Check sheet for the modelled part. Datum: model origin and axes. Units: mm. A direction names the side the tool comes from. Give positions to 0.01 mm unless a question says otherwise; leave off trailing zeros. Write each loop counter-clockwise with the first axis right and the second up, starting at its lowest first coordinate (ties: lowest second). Pieces come first, ordered by that corner, then holes. Notation, with made-up numbers: (64.5, -0.75) - (118.5, -0.75) arc R27 cw to (118.5, 36.25) - close; hole circle Ø2 at (45.25, 27.25). An arc over 180 degrees is marked (long way). Return JSON: item names as keys, results as strings. Group by question number.
```python
from build123d import *

# Parameters (mm, degrees)
SKETCH_1_W           = 17
SKETCH_1_H           = 6
EXTRUDE_1_DEPTH      = 15
EXTRUDE_2_DEPTH      = 6
EXTRUDE_2_DEPTH_BACK = 6
FILLET_4_R           = 1
FILLET_5_R           = 1
FILLET_6_R           = 1


with BuildPart() as part:
    # Эскиз1 → Бобышка-Вытянуть1 (new body)
    with BuildSketch(Plane.XY):
        with BuildLine():
            Line((30, 0), (-30, 0))
            ThreePointArc((-30, 0), (0, -30), (30, 0))
        make_face()
        with Locations((0, -12.426630435)):
            Rectangle(SKETCH_1_W, SKETCH_1_H, mode=Mode.SUBTRACT)
    extrude(amount=EXTRUDE_1_DEPTH)

    # Эскиз6 → Бобышка-Вытянуть2 (add, two sides: drawn at the far end of the back side and taken through both)
    with BuildSketch(Plane(origin=(0, 0, 0), x_dir=(0, 0, -1), z_dir=(1, 0, 0)).offset(-EXTRUDE_2_DEPTH_BACK)):
        Polygon((-14.990436671, -0.00212283), (-14.990436671, 17.99787717), (10.009563329, 17.99787717), (10.009563329, 11.99787717), (-8.498173606, 11.99787717), (-8.498173606, -0.00212283), align=None)
    extrude(amount=EXTRUDE_2_DEPTH + EXTRUDE_2_DEPTH_BACK)

    # Скругление4
    fillet_4_edges = [part.edges().sort_by_distance(p)[0] for p in [
        (-6, 8.998938585, 14.990436671),
    ]]
    fillet(fillet_4_edges, radius=FILLET_4_R)

    # Скругление5
    fillet_5_edges = [part.edges().sort_by_distance(p)[0] for p in [
        (6, 8.998938585, 14.990436671),
        (6, 17.99787717, 2.490436671),
        (-6, 17.99787717, 1.990436671),
        (0.5, 17.99787717, 14.990436671),
        (-5.707106781, 17.99787717, 14.697543453),
    ]]
    fillet(fillet_5_edges, radius=FILLET_5_R)

    # Скругление6
    fillet_6_edges = [part.edges().sort_by_distance(p)[0] for p in [
        (-6, 5.998938585, 8.498173606),
        (0, 11.99787717, 8.498173606),
        (6, 5.998938585, 8.498173606),
        (6, 11.99787717, -0.755694861),
        (-6, 11.99787717, -0.755694861),
    ]]
    fillet(fillet_6_edges, radius=FILLET_6_R)


solid = part.part
```
Item 1: Material ranges on line 1 along Z through (x, y) = (-13, -10); line 2 along X through (y, z) = (14.5, -1); line 3 along Y through (x, z) = (5, -4.75), recorded low to high. Write a range as from..to.
Item 2: Depth check by flat-ended pin: pin 1 (10 mm diameter, centred on x = -4.5, z = -5.5, fed in from -Y); pin 2 (1 mm diameter, centred on x = -1.5, z = 9.5, fed in from -Y); pin 3 (10 mm diameter, centred on x = -23.5, z = 11.5, fed in from -Y); pin 4 (8.5 mm diameter, centred on y = 5, z = -0.5, fed in from +X). Enter the tip coordinate at first touch or a pass-through.
Item 3: Mould release check, pull along X, two halves, no side actions. Record for faces 1 (the face through (-0.66, -29.993, 7.395)), 2 (the face through (0, -8, 15)), 3 (the face through (0, -15.427, 7)): +X half, -X half, draft (parallel to the pull), parting line (faces both ways), or undercut.
Item 4: Section check C-C on y = -11. Record the cut outline in (x, z), plus the area to 3 significant figures.
Item 5: Access from +Z, -Z, +X, -X, +Y, -Y to the whole of each face (thin tool, end or side, straight path). Record for faces 4 (the face through (-8.5, -12, 7)), 5 (the face through (6, 14, 7)), 6 (the face through (0, 15, -10.01)), 7 (the face through (0, 6, 8.498)), 8 (the face through (-6, 14, 7)).
Item 6: Section check A-A on z = 5. Record the cut outline in (x, y), plus the area to 3 significant figures.
Item 7: Section check D-D on z = -2.75. Record the cut outline in (x, y), plus the area to 3 significant figures.
Reply:
{
 "1": {"line 1": "0..15", "line 2": "-6..6", "line 3": "12..18"},
 "2": {"pin 1": "y = 12", "pin 2": "y = -29.98", "pin 3": "y = -23.62", "pin 4": "through"},
 "3": {"face 1": "parting line", "face 2": "draft", "face 3": "undercut"},
 "4": {"outline": "(-27.91, 0) - (-8.5, 0) - (-8.5, 15) - (-27.91, 15) - close; (8.5, 0) - (27.91, 0) - (27.91, 15) - (8.5, 15) - close", "area": "582 mm²"},
 "5": {"face 4": "+Z, -Z", "face 5": "+Z, -Z, +X, +Y", "face 6": "-Z, +X, -X, +Y, -Y", "face 7": "-Z, +X, -X", "face 8": "+Z, -Z, -X, +Y"},
 "6": {"outline": "(-30, 0) arc R30 ccw to (30, 0) - close; (-6, 13) arc R1 ccw to (-5, 12) - (5, 12) arc R1 ccw to (6, 13) - (6, 17) arc R1 ccw to (5, 18) - (-5, 18) arc R1 ccw to (-6, 17) - close; hole (-8.5, -15.43) - (8.5, -15.43) - (8.5, -9.43) - (-8.5, -9.43) - close", "area": "1,380 mm²"},
 "7": {"outline": "(-6, 13) arc R1 ccw to (-5, 12) - (5, 12) arc R1 ccw to (6, 13) - (6, 17) arc R1 ccw to (5, 18) - (-5, 18) arc R1 ccw to (-6, 17) - close", "area": "71.1 mm²"}
}
